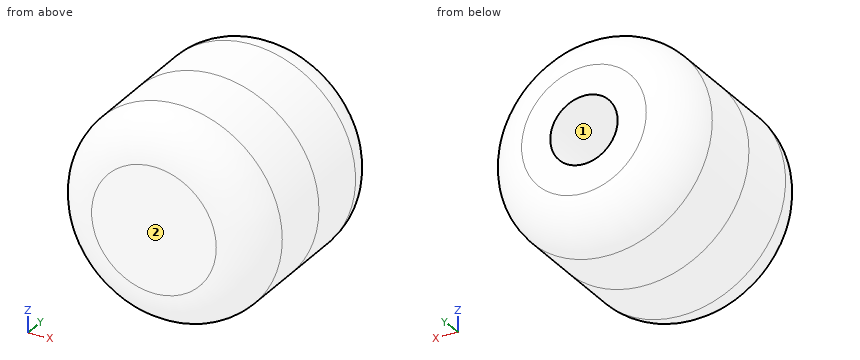
```python
from build123d import *

# Parameters (mm, degrees)
F0_R     = 6.35
F1_DEPTH = 6.35
F2_R     = 6.35
F2_R_2   = 2.0574
F3_DEPTH = 6.35
F4_R     = 2.54


with BuildPart() as f1:
    # F0 (on Front) → F1 (new body)
    with BuildSketch(Plane.XZ):
        Circle(F0_R)
    extrude(amount=F1_DEPTH)

    # F2 (on face) → F3 (join)
    with BuildSketch(Plane(origin=(0, 0, 0), x_dir=(-1, 0, 0), z_dir=(0, 1, 0))):
        Circle(F2_R)
        Circle(F2_R_2, mode=Mode.SUBTRACT)
    extrude(amount=F3_DEPTH)

    # F4
    f4_edges = [f1.edges().sort_by_distance(p)[0] for p in [
        (-6.35, -6.35, 0),
        (6.35, 6.35, 0),
    ]]
    fillet(f4_edges, radius=F4_R)


solid = f1.part
```
Could you check a few things on this model? Use its own coordinates, in mm. Face numbers are marked on the shaded views. Round coordinates to 2 decimals unless told otherwise and drop trailing zeros. Write each loop counter-clockwise with the first axis right and the second up, starting at its lowest first coordinate (ties: lowest second). Pieces come first, ordered by that corner, then holes. Notation, with made-up numbers: M 51,15 L 74,15 A25 ccw 74,39 Z; hole C 29.5,28 d1. An arc over 180 degrees is marked long. Answer in a Markdown table with one row per item. Add a question column.
Q1. Imagine slicing it at C-C (y = 3.25). Please give me the cut outline in (x, z).
Q2. If we mould it in two halves opening along Z, with no side actions, what happens to the marked faces 1 and 2? For each: +Z half, -Z half, draft (parallel to the pull), parting line (faces both ways), or undercut.
Q3. Imagine slicing it at D-D (y = -3). Please give me the cut outline in (x, z), then the cut area to 3 significant figures.
Q4. If I drill on line 1 (Z direction, x = 0, y = 3.5); line 2 (X direction, y = 0.25, z = -1.75); line 3 (Z direction, x = 0, y = 5.25), over which ranges is the centre line in solid material (lowest first)? Write a range as from..to.
Q5. Imagine slicing it at A-A (x = 0). Please give me the cut outline in (y, z).
Q6. Imagine slicing it at B-B (z = 0). Please give me the cut outline in (x, y).
Q7. Will these pins go through, and if not, where does the flat tip stop? pin 1 Ø5 at (y, z) = (3, -3) entering from -X; pin 2 Ø6 at (x, y) = (3, -0.5) entering from +Z; pin 3 Ø1.5 at (x, y) = (-3.5, -2.5) entering from +Z; pin 4 Ø2.5 at (x, z) = (0, 0) entering from +Y.
Values:
| question | item | result |
|---|---|---|
| 1 | outline | C 0,0 d12.7; hole C 0,0 d4.11 |
| 2 | face 1 | undercut |
| 2 | face 2 | draft |
| 3 | outline | C 0,0 d12.7 |
| 3 | area | 127 mm^2 |
| 4 | line 1 | -6.35..-2.06, 2.06..6.35 |
| 4 | line 2 | -6.1..-1.08, 1.08..6.1 |
| 4 | line 3 | -5.9..-2.06, 2.06..5.9 |
| 5 | outline | M -6.35,-3.81 A2.54 ccw -3.81,-6.35 L 3.81,-6.35 A2.54 ccw 6.35,-3.81 L 6.35,-2.06 L 0,-2.06 L 0,2.06 L 6.35,2.06 L 6.35,3.81 A2.54 ccw 3.81,6.35 L -3.81,6.35 A2.54 ccw -6.35,3.81 Z |
| 6 | outline | M -6.35,-3.81 A2.54 ccw -3.81,-6.35 L 3.81,-6.35 A2.54 ccw 6.35,-3.81 L 6.35,3.81 A2.54 ccw 3.81,6.35 L 2.06,6.35 L 2.06,0 L -2.06,0 L -2.06,6.35 L -3.81,6.35 A2.54 ccw -6.35,3.81 Z |
| 7 | pin 1 | x = -6.33 |
| 7 | pin 2 | z = 6.35 |
| 7 | pin 3 | z = 5.72 |
| 7 | pin 4 | y = 0 |
